from build123d import *

# Parameters (mm, degrees)
F0_W      = 187.325
F0_H      = 152.4
F1_DEPTH  = 38.1
F3_D      = 9.5758
F4_DEPTH  = 6.35
F6_DEPTH  = 6.35
F8_D      = 7.9375
F8_DEPTH  = 17.4625
F8_TIP    = 2.3846655818
F10_D     = 7.9375
F10_DEPTH = 17.4625
F10_TIP   = 2.3846655818
F11_D     = 10.3124


with BuildPart() as f1:
    # F0 (on Front) → F1 (new body)
    with BuildSketch(Plane.XZ):
        with Locations((17.3622183502, -12.1438738748)):
            Rectangle(F0_W, F0_H)
        with BuildLine():
            ThreePointArc((73.7470006338, -11.0550622269), (74.2119686187, -12.1775942421), (73.7470006338, -13.3001262572))
            Line((73.7470006338, -13.3001262572), (18.5184254892, -68.5287014018))
            ThreePointArc((18.5184254892, -68.5287014018), (17.3958934741, -68.9936693866), (16.273361459, -68.5287014018))
            Line((16.273361459, -68.5287014018), (-38.9552136856, -13.3001262572))
            ThreePointArc((-38.9552136856, -13.3001262572), (-39.4201816705, -12.1775942421), (-38.9552136856, -11.0550622269))
            Line((-38.9552136856, -11.0550622269), (16.273361459, 44.1735129177))
            ThreePointArc((16.273361459, 44.1735129177), (17.3958934741, 44.6384809025), (18.5184254892, 44.1735129177))
            Line((18.5184254892, 44.1735129177), (73.7470006338, -11.0550622269))
        make_face(mode=Mode.SUBTRACT)
    extrude(amount=F1_DEPTH)

    # F3 (through all)
    with Locations(Plane(origin=(0, 0, 0), x_dir=(1, 0, 0), z_dir=(0, 1, 0))):
        with Locations((-58.8377816498, -25.9561261252), (-58.8377816498, 50.2438738748), (93.5622183502, 50.2438738748), (93.5622183502, -25.9561261252)):
            Hole(F3_D / 2)

    # F2 (on face) → F4 (cut)
    with BuildSketch(Plane.XZ.offset(38.1)):
        with BuildLine():
            Line((-20.9021291893, 15.9782783904), (14.9574931524, 51.8379007322))
            Line((14.9574931524, 51.8379007322), (17.3622183502, 51.8379006441))
            Line((17.3622183502, 51.8379006441), (17.3622183502, 64.0561261252))
            Line((17.3622183502, 64.0561261252), (-37.1623212801, 64.0561261252))
            Line((-37.1623212801, 64.0561261252), (-37.1623212801, 22.7134704812))
            ThreePointArc((-37.1623212801, 22.7134704812), (-31.2823809734, 13.913517934), (-20.9021291893, 15.9782783904))
        make_face()
        with BuildLine():
            Line((17.3622183502, 64.0561261252), (17.3622183502, 51.8379006441))
            Line((17.3622183502, 51.8379006441), (19.8342931524, 51.8379005536))
            Line((19.8342931524, 51.8379005536), (55.6265634353, 16.0456302708))
            ThreePointArc((55.6265634353, 16.0456302708), (66.0068152193, 13.9808698144), (71.8867555261, 22.7808223616))
            Line((71.8867555261, 22.7808223616), (71.8867555261, 64.0561261252))
            Line((71.8867555261, 64.0561261252), (17.3622183502, 64.0561261252))
        make_face()
        with BuildLine():
            Line((19.8340516262, -76.1933300919), (17.3558846933, -76.1930850326))
            Line((17.3558846933, -76.1930850326), (17.354683134, -88.3438738748))
            Line((17.354683134, -88.3438738748), (71.8860174681, -88.3438738748))
            Line((71.8860174681, -88.3438738748), (71.8860174681, -47.1367484316))
            ThreePointArc((71.8860174681, -47.1367484316), (66.0060771614, -38.3367958844), (55.6258253773, -40.4015563408))
            Line((55.6258253773, -40.4015563408), (19.8340516262, -76.1933300919))
        make_face()
        with BuildLine():
            Line((17.354683134, -88.3438738748), (17.3558846933, -76.1930850326))
            Line((17.3558846933, -76.1930850326), (14.9572517743, -76.1928478381))
            Line((14.9572517743, -76.1928478381), (-20.9013891274, -40.3342069364))
            ThreePointArc((-20.9013891274, -40.3342069364), (-31.2816409115, -38.26944648), (-37.1615812182, -47.0693990272))
            Line((-37.1615812182, -47.0693990272), (-37.1615812182, -88.3438738748))
            Line((-37.1615812182, -88.3438738748), (17.354683134, -88.3438738748))
        make_face()
    extrude(amount=-F4_DEPTH, mode=Mode.SUBTRACT)

    # F5 (on face) → F6 (cut)
    with BuildSketch(Plane.XZ):
        with BuildLine():
            Line((15.0345185454, 51.9149261252), (19.7572675809, 51.9149261252))
            Line((19.7572675809, 51.9149261252), (55.6231262594, 16.0490674467))
            ThreePointArc((55.6231262594, 16.0490674467), (66.0033780434, 13.9843069903), (71.8833183502, 22.7842595375))
            Line((71.8833183502, 22.7842595375), (71.8833183502, 64.0561261252))
            Line((71.8833183502, 64.0561261252), (-37.1588803828, 64.0561261252))
            Line((-37.1588803828, 64.0561261252), (-37.1588803828, 22.7169113786))
            ThreePointArc((-37.1588803828, 22.7169113786), (-31.2789400761, 13.9169588314), (-20.898688292, 15.9817192878))
            Line((-20.898688292, 15.9817192878), (15.0345185454, 51.9149261252))
        make_face()
        with BuildLine():
            Line((-37.1588816498, -88.3438738748), (71.8833208084, -88.3438738748))
            Line((71.8833208084, -88.3438738748), (71.8833208084, -47.1394455633))
            ThreePointArc((71.8833208084, -47.1394455633), (66.0033805017, -38.3394930162), (55.6231287176, -40.4042534725))
            Line((55.6231287176, -40.4042534725), (19.7572675809, -76.2701146093))
            Line((19.7572675809, -76.2701146093), (15.0345185454, -76.2701146093))
            Line((15.0345185454, -76.2701146093), (-20.898689559, -40.3369065048))
            ThreePointArc((-20.898689559, -40.3369065048), (-31.2789413431, -38.2721460485), (-37.1588816498, -47.0720985956))
            Line((-37.1588816498, -47.0720985956), (-37.1588816498, -88.3438738748))
        make_face()
    extrude(amount=F6_DEPTH, mode=Mode.SUBTRACT)

    # F8
    with Locations(Plane(origin=(0, 0, -88.3438738748), x_dir=(1, 0, 0), z_dir=(0, 0, -1))):
        with Locations((-42.9627819467, 19.0499955808), (-4.8627819467, 19.0499983719), (77.6872180533, 19.0500044192), (39.5872180533, 19.0500016281)):
            Hole(F8_D / 2, depth=F8_DEPTH)
            with Locations((0, 0, -(F8_DEPTH + F8_TIP / 2))):  # 118° drill point
                Cone(0, F8_D / 2, F8_TIP, mode=Mode.SUBTRACT)

    # F10
    with Locations(Plane.XY.offset(64.0561261252)):
        with Locations((-42.9627810163, -19.05), (-4.8627810163, -19.05), (39.5872189837, -19.05), (77.6872189837, -19.05)):
            Hole(F10_D / 2, depth=F10_DEPTH)
            with Locations((0, 0, -(F10_DEPTH + F10_TIP / 2))):  # 118° drill point
                Cone(0, F10_D / 2, F10_TIP, mode=Mode.SUBTRACT)

    # F11 (through all)
    with Locations(Plane(origin=(0, 0, 0), x_dir=(1, 0, 0), z_dir=(0, 1, 0))):
        with Locations((-58.8377816498, 72.4688738748), (-58.8377816498, 12.1438738748), (-58.8377816498, -48.1811261252), (93.5622183502, -48.1811261252), (93.5622183502, 12.1438738748), (93.5622183502, 72.4688738748)):
            Hole(F11_D / 2)


solid = f1.part
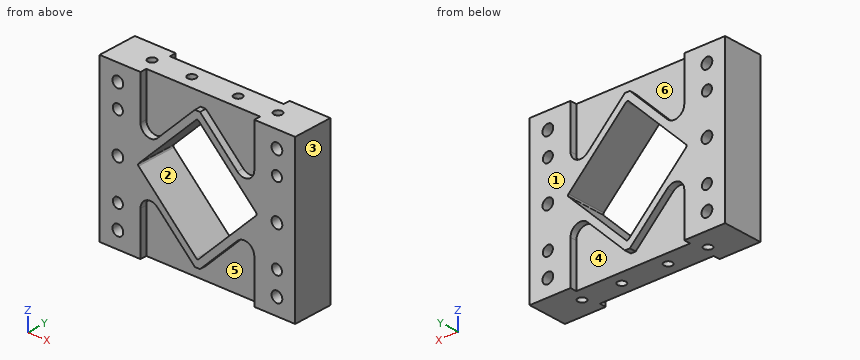
Read the model definition and answer for the solid it produces. Units are mm, in the model's axes. Face numbers are marked on the shaded views. A direction names the side the tool comes from. Give positions to 0.01 mm unless a question says otherwise; leave off trailing zeros. One line per item, written item: value. Start each with the question number.
(1) A tool of negligible diameter and unlimited length cuts with its end or side. For the marked faces 4, 5 and 6, from which of +Z, -Z, +X, -X, +Y, -Y can it reach the whole face along a straight path? Write none if from no direction.
(2) Find the intervals of material crossed by line 1 (Z direction, x = 92, y = -4); line 2 (X direction, y = -35, z = -76.5); line 3 (Z direction, x = 93, y = -28.5), in increasing order.
(3) Flat-ended cylindrical pins translate along their axes: pin 1 Ø10.5 at (x, y) = (-42.96, -19.05) entering from -Z; pin 2 Ø6.5 at (x, y) = (-4.86, -19.05) entering from +Z; pin 3 Ø4 at (x, y) = (17.5, -1.5) entering from +Z; pin 4 Ø1.4 at (x, y) = (18, -3) entering from -Z. Find the tip coordinate at first contact, or state that the pin passes through.
(4) Determine the mould class of the marked faces 1, 2 and 3 for opening direction X: pulls with the +X half, pulls with the -X half, needs draft (parallel to the pull), parting line crosses it, or undercut.
(5) Find section A-A (y = -29.5). Give the number of separate pieces and of enclosed holes in the cut face, plus the area to 3 significant figures.
Results below:
1. face 4: -Z, +Y
1. face 5: -Z, -Y
1. face 6: +Z, +Y
2. line 1: z = -88.34 to -77.38, -67.56 to -54.77, -45.72 to -17.06, -7.23 to 21.43, 30.48 to 43.27, 53.09 to 64.06
2. line 2: x = -76.3 to -62.05, -55.62 to -37.16, 71.89 to 90.35, 96.78 to 111.02
2. line 3: z = -88.34 to -77.59, -67.34 to -55, -45.49 to -17.27, -7.02 to 21.2, 30.71 to 43.06, 53.31 to 64.06
3. pin 1: stops at z = -88.34
3. pin 2: stops at z = 46.16
3. pin 3: stops at z = 51.91
3. pin 4: stops at z = -76.27
4. face 1: needs draft
4. face 2: undercut
4. face 3: pulls with the +X half
5. separate pieces: 1
5. enclosed holes: 11
5. area: 21,200 mm^2
